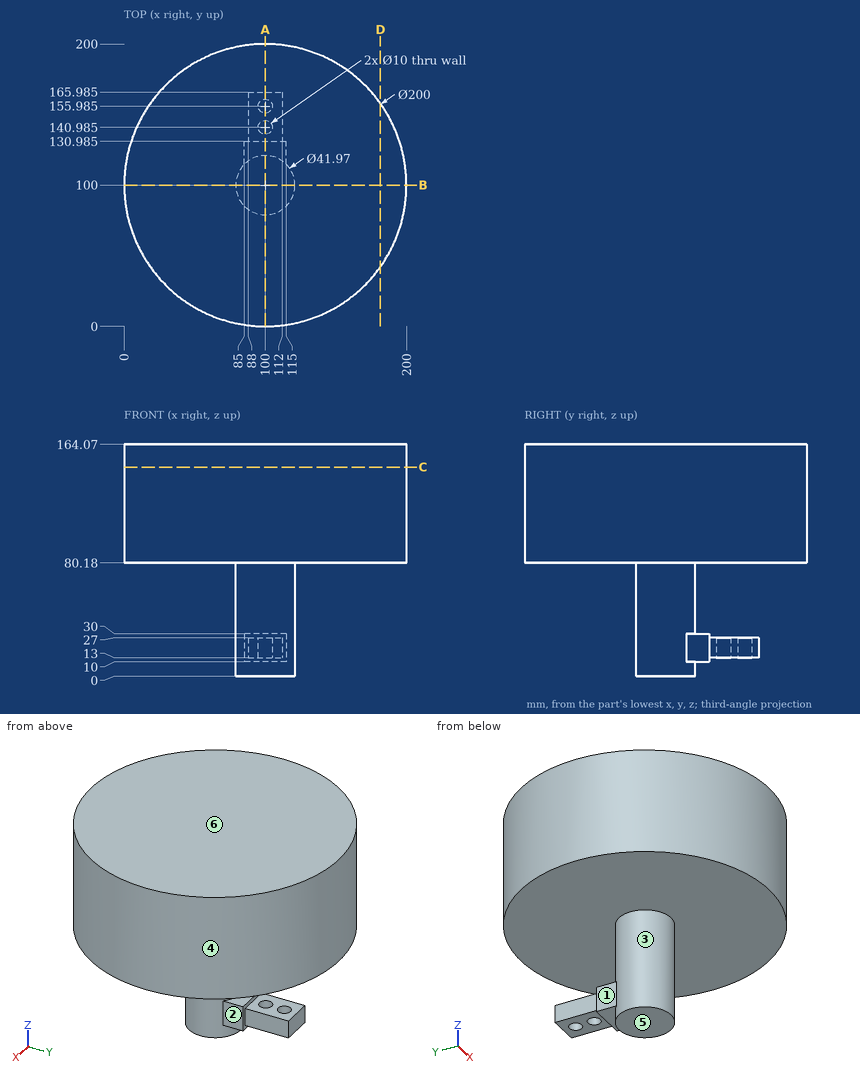
Source: three-view drawing plus pictorial views. Frame: mm from the lowest corner of the part. A direction names the side the tool comes from. Give positions to 0.01 mm unless a question says otherwise; leave off trailing zeros. Write each loop counter-clockwise with the first axis right and the second up, starting at its lowest first coordinate (ties: lowest second). Pieces come first, ordered by that corner, then holes. Notation, with made-up numbers: M 35,35 L 92,35 A23 ccw 92,59 Z; hole C 51.5,-38.5 d11. An arc over 180 degrees is marked long. Use one line per item in the form item = value.
1. Ray query, L1, parallel to Y at x = 100, z = 17.5 (3 decimals); L2, parallel to Z at x = 96.5, y = 146.5; L3, parallel to X at y = 152, z = 17.5. Return the intervals inside material, ascending.
Outcome:
L1 = 79.015 to 135.985, 145.985 to 150.985, 160.985 to 165.985
L2 = 13 to 27, 80.18 to 164.07
L3 = 88 to 96.98, 103.02 to 112
2. Reachability of the marked faces 1 and 2 from +Z, -Z, +X, -X, +Y, -Y: full face, straight path, thin tool, end or side. Return the list, or none.
Outcome:
face_1 = -Z, -X, +Y
face_2 = -Z, +X, +Y
3. Cut plane D-D on x = 181.5. Return loops of the section in (y, z).
Outcome:
outline = M 42.05,80.18 L 157.95,80.18 L 157.95,164.07 L 42.05,164.07 Z
4. First-contact query: P1, Ø11, axis at x = 95.5, z = 18, coming from the +Y side (3 decimals); P2, Ø2, axis at x = 122.5, y = 82, coming from the -Z side; P3, Ø2, axis at x = 130, z = 109, coming from the -Y side; P4, Ø5, axis at x = 97, y = 119.5, coming from the -Z side. Flat tips, straight axial feed; report the tip coordinate or a pass-through.
Outcome:
P1 = 165.985
P2 = 80.18
P3 = 4.3
P4 = 0
5. Cut plane B-B on y = 100. Return loops of the section in (x, z) (3 decimals).
Outcome:
outline = M 0,80.18 L 79.015,80.18 L 79.015,0 L 120.985,0 L 120.985,80.18 L 200,80.18 L 200,164.07 L 0,164.07 Z
6. Cut plane A-A on x = 100. Return loops of the section in (y, z) (3 decimals), and give its area (3 significant figures).
Outcome:
outline = M 0,80.18 L 79.015,80.18 L 79.015,0 L 120.985,0 L 120.985,10 L 130.985,10 L 130.985,13 L 135.985,13 L 135.985,27 L 130.985,27 L 130.985,30 L 120.985,30 L 120.985,80.18 L 200,80.18 L 200,164.07 L 0,164.07 Z; M 145.985,13 L 150.985,13 L 150.985,27 L 145.985,27 Z; M 160.985,13 L 165.985,13 L 165.985,27 L 160.985,27 Z
area = 20,600 mm²
7. Cut plane C-C on z = 148. Return loops of the section in (x, y), and give its area (3 significant figures).
Outcome:
outline = C 100,100 d200
area = 31,400 mm²
8. Mould query, pull axis Z, two halves, no side actions, for the marked faces 3, 4, 5 and 6. Classes: released by +Z, released by -Z, zero draft, split by the parting line, or undercut.
Outcome:
face_3 = undercut
face_4 = zero draft
face_5 = released by -Z
face_6 = released by +Z
